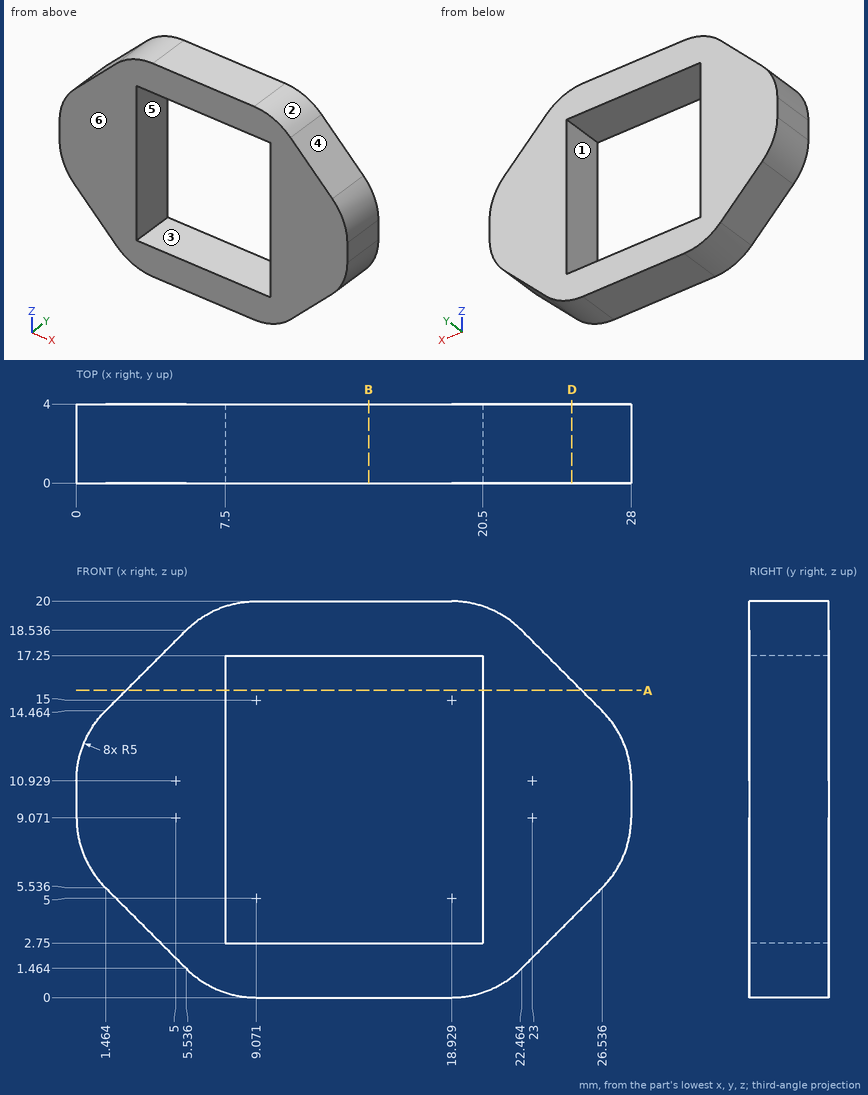
Verification items for this drawing (mm, ordinates from the low corner). A direction names the side the tool comes from. Round coordinates to 2 decimals unless told otherwise and drop trailing zeros. Loops run counter-clockwise (first coordinate to the right, second up) from the corner with the lowest first, then second, coordinate; pieces in that order, holes last. Notation, with made-up numbers: (-17, 13.25) - (35, 13.25) arc R18 ccw to (35, 24.25) - close; hole circle Ø6 at (-3.5, 35). An arc over 180 degrees is marked (long way). Answer as CSV lines item,"result". Start each with the question number.
Item 1: Section check D-D (x = 25). Record the boundary of the cut face in (y, z), and give its area (3 significant figures).
Item 2: Set-up check for the marked faces 1 and 2: record each of +Z, -Z, +X, -X, +Y, -Y from which the full face is reachable in a straight line by a thin tool's end or side.
Item 3: Scan lines: line 1 (Z direction, x = 14.75, y = 2.4); line 2 (X direction, y = 3.6, z = 16.75); line 3 (X direction, y = 1.8, z = 16.5). Record each from-to range of solid material in increasing order. Write a range as [from, to].
Item 4: Section check A-A (z = 15.5). Record the boundary of the cut face in (x, y), and give its area (3 significant figures).
Item 5: Depth check by flat-ended pin: P1, Ø3, axis at x = 17, z = 15, coming from the +Y side; P2, Ø2, axis at y = 1.5, z = 3.5, coming from the +X side; P3, Ø2, axis at y = 1.5, z = 12.5, coming from the -X side; P4, Ø2, axis at y = 2, z = 5, coming from the +X side (1 decimal). Enter the tip coordinate at first touch or a pass-through.
Item 6: Section check B-B (x = 14.75). Record the boundary of the cut face in (y, z), and give its area (3 significant figures).
Item 7: Release check for a two-part mould opening along X. For the marked faces 3, 4, 5 and 6 record: +X half, -X half, draft (parallel to the pull), parting line (faces both ways), or undercut.
Report:
1,outline,"(0, 4) - (4, 4) - (4, 16) - (0, 16) - close"
1,area,"48.0 mm2"
2,face 1,"+Y, -Y"
2,face 2,"+Z, +X, +Y, -Y"
3,line 1,"z = [0, 2.75], [17.25, 20]"
3,line 2,"x = [3.75, 7.5], [20.5, 24.25]"
3,line 3,"x = [3.5, 7.5], [20.5, 24.5]"
4,outline,"(2.5, 0) - (7.5, 0) - (7.5, 4) - (2.5, 4) - close; (20.5, 0) - (25.5, 0) - (25.5, 4) - (20.5, 4) - close"
4,area,"40.0 mm2"
5,P1,"passes through"
5,P2,"stops at x = 25.5"
5,P3,"stops at x = 0.03"
5,P4,"stops at x = 26.9"
6,outline,"(0, 0) - (4, 0) - (4, 2.75) - (0, 2.75) - close; (0, 17.25) - (4, 17.25) - (4, 20) - (0, 20) - close"
6,area,"22.0 mm2"
7,face 3,"undercut"
7,face 4,"+X half"
7,face 5,"undercut"
7,face 6,"draft"
